Verification items for the finished model (mm, model axes). Face numbers are marked on the shaded views. A direction names the side the tool comes from. Coordinates: 2 decimals unless noted, no trailing zeros. Order: outer loops, then holes, each group sorted by start corner. A loop starts at its lowest first (then second) coordinate and runs counter-clockwise, first axis right, second up. Notation, with made-up numbers: (87, 31.5) -> (123, 31.5) arc R15 cw to (123, 52.5) -> close; hole circle Ø8 at (22.25, -5.5). An arc over 180 degrees is marked (long way). Answer as CSV lines item,"result".
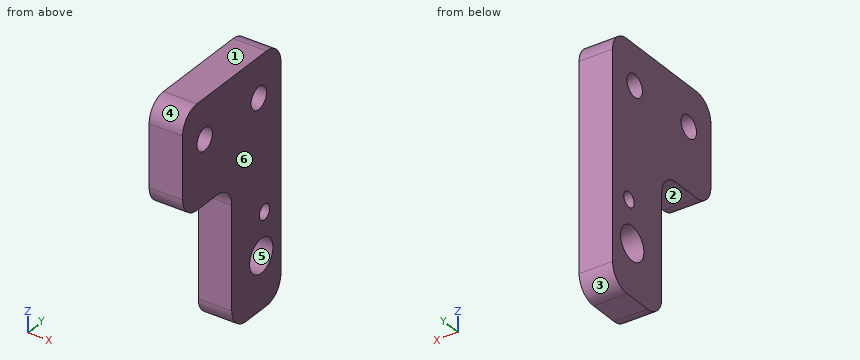
```python
from build123d import *

# Parameters (mm, degrees)
F0_R     = 4.1275
F0_R_2   = 1.8415
F0_R_3   = 2.7305
F1_DEPTH = 8.255
F2_R     = 5.08
F3_R     = 5.08


with BuildPart() as f1:
    # F0 (on Right) → F1 (new body)
    with BuildSketch(Plane.YZ):
        Polygon((-17.399, 0), (0, 0), (0, 60.8), (-34.798, 60.8), (-34.798, 35.4), (-17.399, 35.4), align=None)
        with Locations((-6.9469, 12.8905)):
            Circle(F0_R, mode=Mode.SUBTRACT)
        with Locations((-5.7785, 22.7965)):
            Circle(F0_R_2, mode=Mode.SUBTRACT)
        with Locations((-26.9875, 50.9575)):
            Circle(F0_R_3, mode=Mode.SUBTRACT)
        with Locations((-7.8105, 50.9575)):
            Circle(F0_R_3, mode=Mode.SUBTRACT)
    extrude(amount=F1_DEPTH)

    # F2
    f2_edges = [f1.edges().sort_by_distance(p)[0] for p in [
        (4.1275, 0, 60.8),
    ]]
    fillet(f2_edges, radius=F2_R)

    # F3
    f3_edges = [f1.edges().sort_by_distance(p)[0] for p in [
        (4.1275, 0, 0),
        (4.1275, -17.399, 0),
        (4.1275, -17.399, 35.4),
        (4.1275, -34.798, 35.4),
        (4.1275, -34.798, 60.8),
    ]]
    fillet(f3_edges, radius=F3_R)


solid = f1.part
```
Item 1: Release check for a two-part mould opening along Z. For the marked faces 3, 4, 5 and 6 record: +Z half, -Z half, draft (parallel to the pull), parting line (faces both ways), or undercut.
Answer list:
face 3,"-Z half"
face 4,"+Z half"
face 5,"undercut"
face 6,"draft"
Item 2: Section check A-A, the plane y = -27. Record the boundary of the cut face in (x, z) (3 decimals), plus the area to 3 significant figures.
Answer list:
outline,"(0, 35.4) -> (8.255, 35.4) -> (8.255, 48.227) -> (0, 48.227) -> close; (0, 53.688) -> (8.255, 53.688) -> (8.255, 60.8) -> (0, 60.8) -> close"
area,"165 mm2"
Item 3: Section check B-B, the plane z = 24. Record the boundary of the cut face in (x, y) (3 decimals).
Answer list:
outline,"(0, -17.399) -> (8.255, -17.399) -> (8.255, -7.172) -> (0, -7.172) -> close; (0, -4.385) -> (8.255, -4.385) -> (8.255, 0) -> (0, 0) -> close"
Item 4: Section check D-D, the plane z = 34. Record the boundary of the cut face in (x, y) (3 decimals), plus the area to 3 significant figures.
Answer list:
outline,"(0, -18.977) -> (8.255, -18.977) -> (8.255, 0) -> (0, 0) -> close"
area,"157 mm2"
Item 5: Section check C-C, the plane x = 7. Record the boundary of the cut face in (y, z) (1 decimal).
Answer list:
outline,"(-34.8, 40.5) arc R5.1 ccw to (-29.7, 35.4) -> (-22.5, 35.4) arc R5.1 cw to (-17.4, 30.3) -> (-17.4, 5.1) arc R5.1 ccw to (-12.3, 0) -> (-5.1, 0) arc R5.1 ccw to (0, 5.1) -> (0, 55.7) arc R5.1 ccw to (-5.1, 60.8) -> (-29.7, 60.8) arc R5.1 ccw to (-34.8, 55.7) -> close; hole circle Ø5.5 at (-27, 51); hole circle Ø8.3 at (-6.9, 12.9); hole circle Ø5.5 at (-7.8, 51); hole circle Ø3.7 at (-5.8, 22.8)"
Item 6: Thickness scan on line 1 (Z direction, x = 3, y = -9.5); line 2 (Y direction, x = 4.75, z = 49.5); line 3 (Z direction, x = 6.5, y = -8). Record the ranges inside material, lowest first.
Answer list:
line 1,"0 to 9.65, 16.13 to 48.81, 53.1 to 60.8"
line 2,"-34.8 to -29.3, -24.68 to -10.12, -5.5 to 0"
line 3,"0 to 8.9, 16.88 to 48.23, 53.68 to 60.8"
Item 7: Tool access check on the marked faces 1 and 2. Record the directions out of +Z, -Z, +X, -X, +Y, -Y that give a thin tool (end or side, any length) a straight path to the whole face; none if there is none.
Answer list:
face 1,"+Z, +X, -X, +Y, -Y"
face 2,"-Z, +X, -X, -Y"
Item 8: Depth check by flat-ended pin: pin 1 Ø3.5 at (x, y) = (5.5, -24.5) entering from -Z; pin 2 Ø3 at (x, z) = (7.5, 31) entering from -Y; pin 3 Ø4 at (x, z) = (4.5, 12) entering from -Y. Enter the tip coordinate at first touch or a pass-through.
Answer list:
pin 1,"z = 35.4"
pin 2,"y = -17.89"
pin 3,"y = -17.4"
